```python
from build123d import *

# Parameters (mm, degrees)
SKETCH4_R               = 40
CUT_EXTRUDE2_DEPTH      = 124.198511713
CUT_EXTRUDE2_DEPTH_BACK = 124.198511713


with BuildPart() as part:
    # Sketch3 → Revolve1 (revolve)
    with BuildSketch(Plane.XY):
        Polygon((100, 50), (-100, 50), (-118.198511713, 100), (-123.198511713, 100), (-105, 50), (-105, 0), (105, 0), (105, 50), (123.198511713, 100), (118.198511713, 100), align=None)
    revolve(axis=Axis((160.387463579, 0, 0), (-1, 0, 0)))

    # Sketch4 → Cut-Extrude2 (cut, two sides)
    with BuildSketch(Plane(origin=(0, 0, 0), x_dir=(0, 0, -1), z_dir=(1, 0, 0))) as cut_extrude2_sk:
        Circle(SKETCH4_R)
    extrude(amount=CUT_EXTRUDE2_DEPTH, mode=Mode.SUBTRACT)
    extrude(cut_extrude2_sk.sketch, amount=-CUT_EXTRUDE2_DEPTH_BACK, mode=Mode.SUBTRACT)


solid = part.part
```
Here's how the part is built. I have some questions about the finished solid (model axes, mm). A direction names the side the tool comes from. Give positions to 0.01 mm unless a question says otherwise; leave off trailing zeros. Loops run counter-clockwise (first coordinate to the right, second up) from the corner with the lowest first, then second, coordinate; pieces in that order, holes last. Notation, with made-up numbers: (10, -29) -> (56, -29) arc R19 ccw to (56, -20) -> close; hole circle Ø4 at (9.5, -34). An arc over 180 degrees is marked (long way). Use one line per item in the form item = value. Start each with the question number.
1) For P1, Ø8, axis at x = 80.5, z = 31.5, coming from the +Y side; P2, Ø12, axis at y = 36.5, z = -33.5, coming from the -X side; P3, Ø1.5, axis at y = -48.5, z = -9, coming from the +X side, each with a flat end and sliding along its axis, tell me the tip position at first contact or that it passes through.
2) Which directions (+Z, -Z, +X, -X, +Y, -Y) give clear straight access to the entire face, cutting with the end or side of a thin tool? Please do faces 3 (the face through (105, 22, -34)), 4 (the face through (-105, -22, -34)), 5 (the face through (-101.138, 50.674, -15.958)).
3) Thinking about a two-plate mould opening in Y: for faces 1 (the face through (100.884, 24.192, 46.512)), 2 (the face through (-105.884, -11.365, 51.181)), which applies, +Y half, -Y half, draft (parallel to the pull), parting line (faces both ways), or undercut?
4) Imagine slicing it at C-C (x = -50.5). Please give me the cut outline in (y, z).
5) Please list where these lines run through material, in increasing order: line 1 along Y through (x, z) = (75, 0); line 2 along X through (y, z) = (43, 25).
6) Imagine slicing it at A-A (z = 0). Please give me the cut outline in (x, y).
Check values:
q1.P1 = 41.76
q1.P2 = -107.02
q1.P3 = 105.03
q2.face_3 = +X
q2.face_4 = -X
q2.face_5 = none
q3.face_1 = parting line
q3.face_2 = undercut
q4.outline = circle Ø100 at (0, 0); hole circle Ø80 at (0, 0)
q5.line_1 = -50 to -40, 40 to 50
q5.line_2 = -105 to 105
q6.outline = (-123.2, -100) -> (-118.2, -100) -> (-100, -50) -> (100, -50) -> (118.2, -100) -> (123.2, -100) -> (105, -50) -> (105, -40) -> (-105, -40) -> (-105, -50) -> close; (-123.2, 100) -> (-105, 50) -> (-105, 40) -> (105, 40) -> (105, 50) -> (123.2, 100) -> (118.2, 100) -> (100, 50) -> (-100, 50) -> (-118.2, 100) -> close
